```python
from build123d import *

# Parameters (mm, degrees)
F0_W      = 12.7
F0_H      = 50.8
F1_DEPTH  = 12.7
F2_W      = 6.35
F2_H      = 12.7
F3_DEPTH  = 12.701
F4_R      = 2.794
F5_DEPTH  = 6.351
F6_R      = 4.7625
F7_DEPTH  = 5.08
F8_R      = 2.413
F9_DEPTH  = 9.525
F10_R     = 2.413
F11_DEPTH = 9.525


with BuildPart() as f1:
    # F0 (on Right) → F1 (new body)
    with BuildSketch(Plane.YZ):
        with Locations((-6.35, 0)):
            Rectangle(F0_W, F0_H)
    extrude(amount=F1_DEPTH)

    # F2 (on face) → F3 (cut, through all)
    with BuildSketch(Plane(origin=(0, 0, 0), x_dir=(-1, 0, 0), z_dir=(0, 1, 0))):
        with Locations((-3.175, -6.35)):
            Rectangle(F2_W, F2_H)
    extrude(amount=-F3_DEPTH, mode=Mode.SUBTRACT)

    # F4 (on face) → F5 (cut, through all)
    with BuildSketch(Plane(origin=(6.35, 0, 0), x_dir=(0, -1, 0), z_dir=(-1, 0, 0))):
        with Locations((6.35, -6.35)):
            Circle(F4_R)
    extrude(amount=-F5_DEPTH, mode=Mode.SUBTRACT)

    # F6 (on face) → F7 (cut)
    with BuildSketch(Plane.YZ.offset(12.7)):
        with Locations((-6.35, -6.35)):
            Circle(F6_R)
    extrude(amount=-F7_DEPTH, mode=Mode.SUBTRACT)

    # F8 (on face) → F9 (cut)
    with BuildSketch(Plane.XY.offset(25.4)):
        with Locations((6.35, -6.35)):
            Circle(F8_R)
    extrude(amount=-F9_DEPTH, mode=Mode.SUBTRACT)

    # F10 (on face) → F11 (cut)
    with BuildSketch(Plane(origin=(0, 0, -25.4), x_dir=(1, 0, 0), z_dir=(0, 0, -1))):
        with Locations((6.35, 6.35)):
            Circle(F10_R)
    extrude(amount=-F11_DEPTH, mode=Mode.SUBTRACT)


solid = f1.part
```
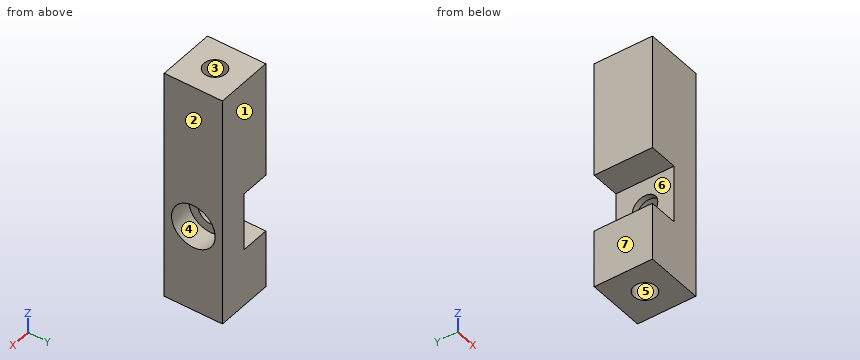
CAD build for the part. Positions are in the model's coordinates, mm. Face numbers are marked on the shaded views. A direction names the side the tool comes from. Round coordinates to 2 decimals unless told otherwise and drop trailing zeros. Order: outer loops, then holes, each group sorted by start corner. A loop starts at its lowest first (then second) coordinate and runs counter-clockwise, first axis right, second up. Notation, with made-up numbers: (60, -12.5) - (87, -12.5) arc R28 cw to (87, 10.5) - close; hole circle Ø3 at (78.5, -35.75). An arc over 180 degrees is marked (long way). Answer in a Markdown table with one row per item. Add a question column.
(1) Mould opens along Y. For the marked faces 1, 2, 3 and 4 say: +Y half, -Y half, draft (parallel to the pull), parting line (faces both ways), or undercut.
(2) 3-axis set-ups, long thin cutter, end or side, ignore diameter. For the marked faces 5, 6 and 7: which of +Z, -Z, +X, -X, +Y, -Y reach the whole face in a straight line?
(3) Band-saw the part on A-A on z = -6.35. List the corners of the cut face in (x, y).
(4) Band-saw the part on C-C on x = 1. List the corners of the cut face in (y, z).
(5) Drop flat-ended pins along their axis: pin 1 Ø6.5 at (y, z) = (-6.35, -6.35) entering from +X; pin 2 Ø4 at (x, y) = (6.35, -6.35) entering from +Z (3 decimals). Give the stop position or say it passes through.
(6) Probe L1, parallel to X at y = -6.35, z = -22.25; L2, parallel to Z at x = 7.1, y = -6.35 (3 decimals); L3, parallel to Z at x = 1.75, y = -5. List the from-to ranges inside material, lowest first. Write a range as [from, to].
Data:
| question | item | result |
|---|---|---|
| 1 | face 1 | +Y half |
| 1 | face 2 | draft |
| 1 | face 3 | undercut |
| 1 | face 4 | undercut |
| 2 | face 5 | -Z |
| 2 | face 6 | -X, +Y, -Y |
| 2 | face 7 | +Z, -Z, -X, +Y, -Y |
| 3 | outline | (6.35, -12.7) - (12.7, -12.7) - (12.7, -11.11) - (7.62, -11.11) - (7.62, -9.14) - (6.35, -9.14) - close; (6.35, -3.56) - (7.62, -3.56) - (7.62, -1.59) - (12.7, -1.59) - (12.7, 0) - (6.35, 0) - close |
| 4 | outline | (-12.7, -25.4) - (0, -25.4) - (0, -12.7) - (-12.7, -12.7) - close; (-12.7, 0) - (0, 0) - (0, 25.4) - (-12.7, 25.4) - close |
| 5 | pin 1 | stops at x = 7.62 |
| 5 | pin 2 | stops at z = 15.875 |
| 6 | L1 | x = [0, 3.94], [8.76, 12.7] |
| 6 | L2 | z = [-15.875, -9.144], [-3.556, 15.875] |
| 6 | L3 | z = [-25.4, -12.7], [0, 25.4] |
